The model under review builds one solid part; all positions refer to its coordinate system, in mm. Face numbers are marked on the shaded views. A direction names the side the tool comes from. Give positions to 0.01 mm unless a question says otherwise; leave off trailing zeros. Loops run counter-clockwise (first coordinate to the right, second up) from the corner with the lowest first, then second, coordinate; pieces in that order, holes last. Notation, with made-up numbers: (65, -34.75) - (82, -34.75) arc R27 ccw to (82, -18.75) - close; hole circle Ø1 at (54, -13). An arc over 180 degrees is marked (long way). Answer as a JSON object with one key per item and string values.
from build123d import *

# Parameters (mm, degrees)
SKETCH_1_W           = 38.3
SKETCH_1_H           = 32
EXTRUDE_1_DEPTH      = 2
EXTRUDE_2_DEPTH      = 75
SKETCH_9_R           = 1.35
CUT_EXTRUDE_5_DEPTH  = 33
SKETCH_10_W          = 15.3
SKETCH_10_H          = 52
CUT_EXTRUDE_6_DEPTH  = 33
SKETCH_11_W          = 28.3
SKETCH_11_H          = 22
CUT_EXTRUDE_7_DEPTH  = 78
SKETCH_13_W          = 18
SKETCH_13_H          = 57
CUT_EXTRUDE_8_DEPTH  = 39.3
SKETCH_14_W          = 5
SKETCH_14_H          = 2
CUT_EXTRUDE_9_DEPTH  = 33
EXTRUDE_3_DEPTH      = 4
EXTRUDE_4_DEPTH      = 4
SKETCH_19_W          = 8
SKETCH_19_H          = 45.4
CUT_EXTRUDE_10_DEPTH = 4
SKETCH_20_W          = 40.713744441
SKETCH_20_H          = 41.376466264
CUT_EXTRUDE_11_DEPTH = 59


with BuildPart() as part:
    # Эскиз1 → Бобышка-Вытянуть1 (new body)
    with BuildSketch(Plane(origin=(0, 0, 0), x_dir=(1, 0, 0), z_dir=(0, 1, 0))):
        Rectangle(SKETCH_1_W, SKETCH_1_H)
    extrude(amount=EXTRUDE_1_DEPTH)

    # Эскиз2 → Бобышка-Вытянуть2 (add)
    with BuildSketch(Plane(origin=(0, 2, 0), x_dir=(1, 0, 0), z_dir=(0, 1, 0))):
        Polygon((-19.15, 16), (19.15, 16), (19.15, -16), (-19.15, -16), (-19.15, -14), (17.15, -14), (17.15, 14), (-19.15, 14), align=None)
    extrude(amount=EXTRUDE_2_DEPTH)

    # Эскиз9 → Вырез-Вытянуть5 (cut, through all)
    with BuildSketch(Plane.XY.offset(16)):
        with Locations((-13.15, 69)):
            Circle(SKETCH_9_R)
        with Locations((-13.15, 10)):
            Circle(SKETCH_9_R)
    extrude(amount=-CUT_EXTRUDE_5_DEPTH, mode=Mode.SUBTRACT)

    # Эскиз10 → Вырез-Вытянуть6 (cut, through all)
    with BuildSketch(Plane.XY.offset(16)):
        with Locations((3.5, 36)):
            Rectangle(SKETCH_10_W, SKETCH_10_H)
    extrude(amount=-CUT_EXTRUDE_6_DEPTH, mode=Mode.SUBTRACT)

    # Эскиз11 → Вырез-Вытянуть7 (cut, through all)
    with BuildSketch(Plane.XZ):
        Rectangle(SKETCH_11_W, SKETCH_11_H)
    extrude(amount=-CUT_EXTRUDE_7_DEPTH, mode=Mode.SUBTRACT)

    # Эскиз13 → Вырез-Вытянуть8 (cut, through all)
    with BuildSketch(Plane(origin=(19.15, 0, 0), x_dir=(0, 0, -1), z_dir=(1, 0, 0))):
        with Locations((0, 38.5)):
            Rectangle(SKETCH_13_W, SKETCH_13_H)
    extrude(amount=-CUT_EXTRUDE_8_DEPTH, mode=Mode.SUBTRACT)

    # Эскиз14 → Вырез-Вытянуть9 (cut, through all)
    with BuildSketch(Plane(origin=(0, 0, -16), x_dir=(-1, 0, 0), z_dir=(0, 0, -1))):
        with Locations((-11.65, 71)):
            Rectangle(SKETCH_14_W, SKETCH_14_H)
        with Locations((1.65, 71)):
            Rectangle(SKETCH_14_W, SKETCH_14_H)
    extrude(amount=-CUT_EXTRUDE_9_DEPTH, mode=Mode.SUBTRACT)

    # Эскиз16 → Бобышка-Вытянуть3 (add)
    with BuildSketch(Plane.XY.offset(16)):
        Polygon((-19.15, 0), (-4.15, 0), (-4.15, 19.8), (-19.15, 19.8), (-19.15, 16.8), (-7.15, 16.8), (-7.15, 3.2), (-19.15, 3.2), align=None)
    extrude_3 = extrude(amount=EXTRUDE_3_DEPTH)

    # Зеркальное отражение1: Бобышка-Вытянуть3 across plane
    add(extrude_3.mirror(Plane.XY))

    # Эскиз18 → Бобышка-Вытянуть4 (add)
    with BuildSketch(Plane.XY.offset(16)):
        Polygon((-19.15, 62.2), (-19.15, 59), (-4.15, 59), (-4.15, 77), (-19.15, 77), (-19.15, 75.8), (-7.15, 75.8), (-7.15, 62.2), align=None)
    extrude_4 = extrude(amount=EXTRUDE_4_DEPTH)

    # Зеркальное отражение2: Бобышка-Вытянуть4 across plane
    add(extrude_4.mirror(Plane.XY))

    # Эскиз19 → Вырез-Вытянуть10 (cut)
    with BuildSketch(Plane.XY.offset(20)):
        with Locations((-15.15, 39.5)):
            Rectangle(SKETCH_19_W, SKETCH_19_H)
    extrude(amount=-CUT_EXTRUDE_10_DEPTH, mode=Mode.SUBTRACT)

    # Эскиз20 → Вырез-Вытянуть11 (cut)
    with BuildSketch(Plane.XZ):
        with Locations((1.20687222, -0.688233132)):
            Rectangle(SKETCH_20_W, SKETCH_20_H)
    extrude(amount=-CUT_EXTRUDE_11_DEPTH, mode=Mode.SUBTRACT)


solid = part.part
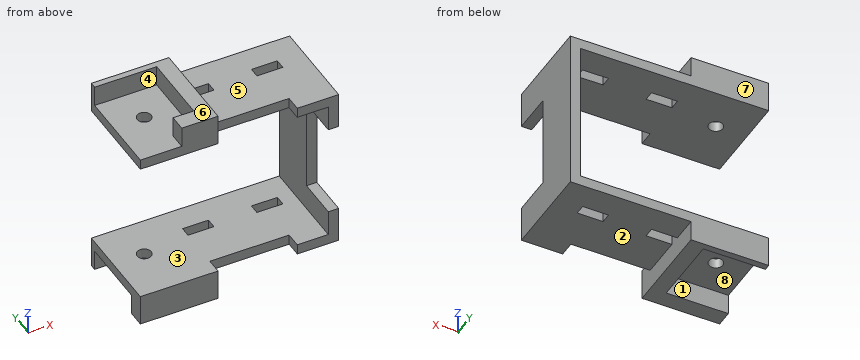
Q1. Consider section A-A, the plane x = -13.15. State the section outline as (y, z) points, plus the area to 3 significant figures.
Results:
{"outline": "(59, -20) - (62.2, -20) - (62.2, -16) - (67.65, -16) - (67.65, -14) - (59, -14) - close; (59, 14) - (67.65, 14) - (67.65, 16) - (59, 16) - close; (70.35, -16) - (75.8, -16) - (75.8, -20) - (77, -20) - (77, -14) - (70.35, -14) - close; (70.35, 14) - (77, 14) - (77, 20) - (75.8, 20) - (75.8, 16) - (70.35, 16) - close", "area": "83.6 mm^2"}
Q2. Consider section B-B, the plane y = 61. State the section outline as (x, z) points, plus the area to 3 significant figures.
Results:
{"outline": "(-19.15, -20) - (-4.15, -20) - (-4.15, -14) - (-19.15, -14) - close; (-19.15, 14) - (-4.15, 14) - (-4.15, 20) - (-11.15, 20) - (-11.15, 16) - (-19.15, 16) - close; (11.15, -16) - (19.15, -16) - (19.15, -9) - (17.15, -9) - (17.15, -14) - (11.15, -14) - close; (11.15, 14) - (17.15, 14) - (17.15, 9) - (19.15, 9) - (19.15, 16) - (11.15, 16) - close", "area": "200 mm^2"}
Q3. Consider section C-C, the plane y = 73. State the section outline as (x, z) points, plus the area to 3 significant figures.
Results:
{"outline": "(-19.15, -16) - (-7.15, -16) - (-7.15, -20) - (-4.15, -20) - (-4.15, -16) - (19.15, -16) - (19.15, 16) - (-4.15, 16) - (-4.15, 20) - (-7.15, 20) - (-7.15, 16) - (-19.15, 16) - (-19.15, 14) - (17.15, 14) - (17.15, -14) - (-19.15, -14) - close", "area": "233 mm^2"}
Q4. Consider section D-D, the plane y = 68.25. State the section outline as (x, z) points, plus the area to 3 significant figures.
Results:
{"outline": "(-19.15, -16) - (-14.27, -16) - (-14.27, -14) - (-19.15, -14) - close; (-19.15, 14) - (-14.27, 14) - (-14.27, 16) - (-19.15, 16) - close; (-12.03, -16) - (-7.15, -16) - (-7.15, -20) - (-4.15, -20) - (-4.15, -16) - (19.15, -16) - (19.15, 16) - (-4.15, 16) - (-4.15, 20) - (-7.15, 20) - (-7.15, 16) - (-12.03, 16) - (-12.03, 14) - (17.15, 14) - (17.15, -14) - (-12.03, -14) - close", "area": "224 mm^2"}
Q5. For the marked faces 1, 2, 3, 4 and 5, list the 3-axis set-ups (+Z, -Z, +X, -X, +Y, -Y) from which the entire face can be reached by the end or side of a thin tool; tool diameter is ignored.
Results:
{"face 1": "-Z, -X", "face 2": "-Z, +X, +Y, -Y", "face 3": "-X, +Y, -Y", "face 4": "+Z, -X", "face 5": "+Z, +X, +Y, -Y"}
Q6. Clearance check with flat-ended pins moving along their axes: pin 1 Ø2 at (x, z) = (-1, 15) entering from -Y; pin 2 Ø2 at (x, z) = (-14.5, 17.5) entering from -Y; pin 3 Ø3 at (x, y) = (-13.15, 69) entering from -Z. State where each tip first meets the part, or that it passes through.
Results:
{"pin 1": "stops at y = 62", "pin 2": "stops at y = 75.8", "pin 3": "stops at z = -16"}
Q7. The part is to be moulded in two halves that separate along Y. For the marked faces 6, 7 and 8, say which applies: +Y half, -Y half, draft (parallel to the pull), parting line (faces both ways), or undercut.
Results:
{"face 6": "draft", "face 7": "+Y half", "face 8": "undercut"}
Q8. To check wall thickness, follow probe 1 along Z at (x, y) = (-3, 68.75); probe 2 along Y at (x, z) = (-13.15, -15.1); probe 3 along X at (y, z) = (69, 15.3). State the ranges of each line that lie inside material, in increasing order. Write a range as [from, to].
Results:
{"probe 1": "z = [-16, -14], [14, 16]", "probe 2": "y = [59, 67.65], [70.35, 77]", "probe 3": "x = [-19.15, -14.5], [-11.8, 19.15]"}
